Work out the finished part from the listing and answer in its coordinate system (mm). Face numbers are marked on the shaded views. A direction names the side the tool comes from. Round coordinates to 2 decimals unless told otherwise and drop trailing zeros. Order: outer loops, then holes, each group sorted by start corner. A loop starts at its lowest first (then second) coordinate and runs counter-clockwise, first axis right, second up.
from build123d import *

# Parameters (mm, degrees)
SKETCH1_R           = 5.75
SKETCH1_R_2         = 2.75
BOSS_EXTRUDE1_DEPTH = 4
SKETCH1_3_R         = 5.75
SKETCH1_3_R_2       = 1.7
SKETCH1_3_R_3       = 2.75
BOSS_EXTRUDE2_DEPTH = 3
FILLET1_R           = 3
FILLET2_R           = 1


with BuildPart() as part:
    # Sketch1 → Boss-Extrude1 (new body)
    with BuildSketch(Plane(origin=(0, 0, 0), x_dir=(1, 0, 0), z_dir=(0, 1, 0))):
        with Locations(Location((0, 0, 0), (0, 0, 270))):
            Circle(SKETCH1_R)
        with Locations(Location((0, 0, 0), (0, 0, 270))):
            Circle(SKETCH1_R_2, mode=Mode.SUBTRACT)
    extrude(amount=BOSS_EXTRUDE1_DEPTH)

    # Sketch1_3 → Boss-Extrude2 (add)
    with BuildSketch(Plane(origin=(0, 0, 0), x_dir=(1, 0, 0), z_dir=(0, 1, 0))):
        with BuildLine():
            ThreePointArc((-20, 15), (-18.535533906, 18.535533906), (-15, 20))
            Line((-15, 20), (15, 20))
            ThreePointArc((15, 20), (18.535533906, 18.535533906), (20, 15))
            Line((20, 15), (20, -15))
            ThreePointArc((20, -15), (18.535533906, -18.535533906), (15, -20))
            Line((15, -20), (-15, -20))
            ThreePointArc((-15, -20), (-18.535533906, -18.535533906), (-20, -15))
            Line((-20, -15), (-20, 15))
        make_face()
        with Locations(Location((0, 0, 0), (0, 0, 270))):
            Circle(SKETCH1_3_R, mode=Mode.SUBTRACT)
        with Locations(Location((15, -15, 0), (0, 0, 270))):
            Circle(SKETCH1_3_R_2, mode=Mode.SUBTRACT)
        with Locations(Location((15, 15, 0), (0, 0, 270))):
            Circle(SKETCH1_3_R_2, mode=Mode.SUBTRACT)
        with Locations(Location((-15, 15, 0), (0, 0, 270))):
            Circle(SKETCH1_3_R_2, mode=Mode.SUBTRACT)
        with Locations(Location((-15, -15, 0), (0, 0, 270))):
            Circle(SKETCH1_3_R_2, mode=Mode.SUBTRACT)
        with Locations(Location((0, 0, 0), (0, 0, 270))):
            Circle(SKETCH1_3_R)
        with Locations(Location((0, 0, 0), (0, 0, 270))):
            Circle(SKETCH1_3_R_3, mode=Mode.SUBTRACT)
    extrude(amount=-BOSS_EXTRUDE2_DEPTH)

    # Fillet1
    fillet1_edges = [part.edges().sort_by_distance(p)[0] for p in [
        (0, 0, -5.75),
    ]]
    fillet(fillet1_edges, radius=FILLET1_R)

    # Fillet2
    fillet2_edges = [part.edges().sort_by_distance(p)[0] for p in [
        (18.535533906, 0, 18.535533906),
        (-18.535533906, 0, 18.535533906),
        (-20, 0, 0),
        (0, 0, 20),
        (20, 0, 0),
        (-18.535533906, 0, -18.535533906),
        (0, 0, -20),
        (18.535533906, 0, -18.535533906),
    ]]
    fillet(fillet2_edges, radius=FILLET2_R)


solid = part.part
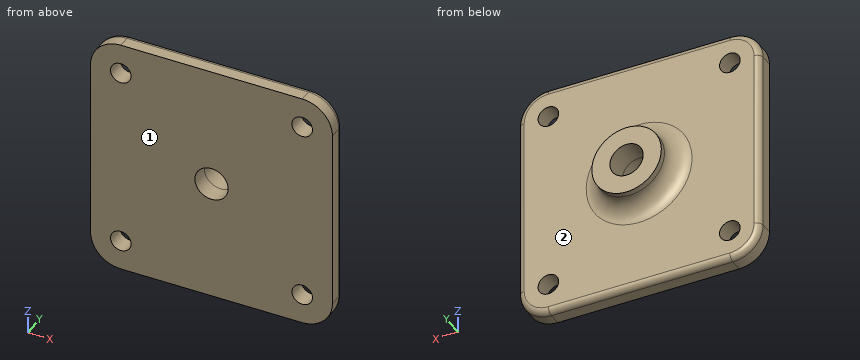
Item 1: Find section A-A (z = 0). Write down the section's boundary in (x, y), plus the area to 3 significant figures.
Item 2: Given pin 1 (4.5 mm diameter, centred on x = 15, z = -15, fed in from +Y); pin 2 (2 mm diameter, centred on x = 15, z = 15, fed in from +Y); pin 3 (3 mm diameter, centred on x = -4.5, y = 3, fed in from +Z); pin 4 (10 mm diameter, centred on x = 5, z = 10.5, fed in from +Y), each flat-ended and moving along its own axis, determine where each tip first touches the part or whether it passes through.
Item 3: Find section B-B (x = -10.5). Write down the section's boundary in (y, z).
Item 4: Find section D-D (y = 3.5). Write down the section's boundary in (x, z).
Item 5: Find section C-C (z = 10.5). Write down the section's boundary in (x, y), plus the area to 3 significant figures.
Item 6: Find the intervals of material crossed by line 1 along X through (y, z) = (-1.1, -15); line 2 along X through (y, z) = (-1.25, -14.5); line 3 along Y through (x, z) = (-17.5, 4.5), in increasing order.
Item 7: A tool of negligible diameter and unlimited length cuts with its end or side. For the marked faces 1 and 2, from which of +Z, -Z, +X, -X, +Y, -Y can it reach the whole face along a straight path? Write none if from no direction.
Model answer:
1. outline: (-20, -3) - (-2.75, -3) - (-2.75, 4) - (-5.75, 4) - (-5.75, 3) arc R3 cw to (-8.75, 0) - (-19, 0) arc R1 ccw to (-20, -1) - close; (2.75, -3) - (20, -3) - (20, -1) arc R1 ccw to (19, 0) - (8.75, 0) arc R3 cw to (5.75, 3) - (5.75, 4) - (2.75, 4) - close
1. area: 131 mm2
2. pin 1: stops at y = 0
2. pin 2: passes through
2. pin 3: stops at z = 4.91
2. pin 4: stops at y = 0.88
3. outline: (-3, -20) - (-1, -20) arc R1 ccw to (0, -19) - (0, 19) arc R1 ccw to (-1, 20) - (-3, 20) - close
4. outline: circle Ø11.5 at (0, 0); hole circle Ø5.5 at (0, 0)
5. outline: (-20, -3) - (20, -3) - (20, -1) arc R1 ccw to (19, 0) - (-19, 0) arc R1 ccw to (-20, -1) - close
5. area: 120 mm2
6. line 1: x = -20 to -16.7, -13.3 to 13.3, 16.7 to 20
6. line 2: x = -20 to -16.62, -13.38 to 13.38, 16.62 to 20
6. line 3: y = -3 to 0
7. face 1: +Z, -Z, +X, -X, -Y
7. face 2: +Y
